from build123d import *

# Parameters (mm, degrees)
F2_DEPTH = 500
F3_DEPTH = 50


with BuildPart() as f2:
    # F0 (on Right) → F2 (new body, symmetric)
    with BuildSketch(Plane.YZ):
        with BuildLine():
            Line((325, -15), (325, 15))
            Line((325, 15), (-320, 15))
            ThreePointArc((-320, 15), (-323.5355339059, 13.5355339059), (-325, 10))
            Line((-325, 10), (-325, -10))
            ThreePointArc((-325, -10), (-323.5355339059, -13.5355339059), (-320, -15))
            Line((-320, -15), (325, -15))
        make_face()
    extrude(amount=F2_DEPTH, both=True)

    # F1 (on Top) → F3 (intersect, symmetric)
    with BuildSketch(Plane.XY):
        Polygon((-377.2004181072, 57.5629813311), (-222.5983966751, -519.420954832), (453.5497866996, -338.2480150228), (298.9477652675, 238.7359211403), align=None)
    extrude(amount=F3_DEPTH, both=True, mode=Mode.INTERSECT)


solid = f2.part
Verification items for the finished model (mm, model axes). Round coordinates to 2 decimals unless told otherwise and drop trailing zeros. Write each loop counter-clockwise with the first axis right and the second up, starting at its lowest first coordinate (ties: lowest second). Pieces come first, ordered by that corner, then holes.
(1) Section check B-B (x = -11). Enter the section's corners in (y, z), plus the area to 3 significant figures.
Returned:
outline: (-325, -10) arc R5 ccw to (-320, -15) - (155.69, -15) - (155.69, 15) - (-320, 15) arc R5 ccw to (-325, 10) - close
area: 14,400 mm2
(2) Section check C-C (y = 98). Enter the section's corners in (x, z), plus the area to 3 significant figures.
Returned:
outline: (-226.29, -15) - (336.66, -15) - (336.66, 15) - (-226.29, 15) - close
area: 16,900 mm2
(3) Section check D-D (x = 185.5). Enter the section's corners in (y, z).
Returned:
outline: (-325, -10) arc R5 ccw to (-320, -15) - (208.34, -15) - (208.34, 15) - (-320, 15) arc R5 ccw to (-325, 10) - close
(4) Section check A-A (z = 4.5). Enter the section's corners in (x, y).
Returned:
outline: (-377.2, 57.56) - (-274.69, -325) - (450, -325) - (298.95, 238.74) - close
(5) Depth check by flat-ended pin: pin 1 Ø5 at (y, z) = (-81.5, 6) entering from -X; pin 2 Ø4 at (y, z) = (87, 7) entering from +X; pin 3 Ø3 at (y, z) = (-235.5, -5) entering from +X. Enter the tip coordinate at first touch or a pass-through.
Returned:
pin 1: stops at x = -340.61
pin 2: stops at x = 340.14
pin 3: stops at x = 426.42
(6) Material ranges on line 1 (Y direction, x = -235, z = 5); line 2 (X direction, y = 53.5, z = 6); line 3 (Y direction, x = -166, z = 11.5), recorded low to high.
Returned:
line 1: y = -325 to 95.67
line 2: x = -376.11 to 348.58
line 3: y = -324.77 to 114.15
